Geometry: final body of the model. Coordinates: model frame, mm. Give positions to 0.01 mm unless a question says otherwise; leave off trailing zeros. Loops run counter-clockwise (first coordinate to the right, second up) from the corner with the lowest first, then second, coordinate; pieces in that order, holes last. Notation, with made-up numbers: (81, 53) -> (133, 53) arc R31 ccw to (133, 81) -> close; hole circle Ø1 at (58, -35.75). An arc over 180 degrees is marked (long way). One line per question, with ' | ' between items. Start each with the question number.
Item 1: Section D-D on z = -2.5. Return loops of the section in (x, y), then the cut area to 3 significant figures.
Item 2: Material intervals for line 1 along Y through (x, z) = (0, -2.4); line 2 along X through (y, z) = (2.5, -0.05); line 3 along X through (y, z) = (1, -0.35), sorted ascending. Write a range as [from, to].
Item 3: Section C-C on z = -0.25. Return loops of the section in (x, y).
Item 4: Pin query (flat end, axial travel): P1, Ø2.5, axis at x = 14, y = 0, coming from the -Z side. Return the tip coordinate at first contact, or that it passes through.
Item 5: Section B-B on x = 18. Return loops of the section in (y, z), then the cut area to 3 significant figures.
Item 6: Mould query, pull axis Y, two halves, no side actions, for faces 1 (the flat face through (21, 0, -1)), 2 (the cylindrical face through (16.62, 0.44, -1.52)), 3 (the cylindrical face through (-2.715, -3.699, -1.521)), 4 (the cylindrical face through (12.661, -0.555, -1.521)). Classes: released by +Y, released by -Y, zero draft, split by the parting line, or undercut.
Item 7: Section A-A on y = -1. Return loops of the section in (x, z).
from build123d import *

# Parameters (mm, degrees)
F0_W     = 6
F0_H     = 8
F0_W_2   = 12
F1_DEPTH = 3
F2_D     = 2.9
F4_D     = 2.3
F5_R     = 1


with BuildPart() as f1:
    # F0 (on Top) → F1 (new body)
    with BuildSketch(Plane.XY):
        Rectangle(F0_W, F0_H)
        with Locations((9, 0)):
            Rectangle(F0_W_2, F0_H)
        with Locations((18, 0)):
            Rectangle(F0_W, F0_H)
    extrude(amount=-F1_DEPTH)

    # F2 (through all)
    with Locations(Plane.XY):
        with Locations((0, 0), (4, 0), (14, 0), (18, 0)):
            Hole(F2_D / 2)

    # F4 (through all)
    with Locations(Plane.XZ.offset(4)):
        with Locations((9, 0)):
            Hole(F4_D / 2)

    # F5
    f5_edges = [f1.edges().sort_by_distance(p)[0] for p in [
        (-3, -4, -1.5),
        (21, -4, -1.5),
        (21, 4, -1.5),
        (-3, 4, -1.5),
    ]]
    fillet(f5_edges, radius=F5_R)


solid = f1.part
Result sheet:
1) outline: (-3, -3) arc R1 ccw to (-2, -4) -> (20, -4) arc R1 ccw to (21, -3) -> (21, 3) arc R1 ccw to (20, 4) -> (-2, 4) arc R1 ccw to (-3, 3) -> close; hole circle Ø2.9 at (0, 0); hole circle Ø2.9 at (4, 0); hole circle Ø2.9 at (14, 0); hole circle Ø2.9 at (18, 0) | area: 165 mm²
2) line 1: y = [-4, -1.45], [1.45, 4] | line 2: x = [-3, 7.85], [10.15, 21] | line 3: x = [-3, -1.05], [1.05, 2.95], [5.05, 7.9], [10.1, 12.95], [15.05, 16.95], [19.05, 21]
3) outline: (-3, -3) arc R1 ccw to (-2, -4) -> (7.88, -4) -> (7.88, 4) -> (-2, 4) arc R1 ccw to (-3, 3) -> close; (10.12, -4) -> (20, -4) arc R1 ccw to (21, -3) -> (21, 3) arc R1 ccw to (20, 4) -> (10.12, 4) -> close; hole circle Ø2.9 at (0, 0); hole circle Ø2.9 at (4, 0); hole circle Ø2.9 at (14, 0); hole circle Ø2.9 at (18, 0)
4) P1: passes through
5) outline: (-4, -3) -> (-1.45, -3) -> (-1.45, 0) -> (-4, 0) -> close; (1.45, -3) -> (4, -3) -> (4, 0) -> (1.45, 0) -> close | area: 15.3 mm²
6) face 1: zero draft | face 2: undercut | face 3: released by -Y | face 4: undercut
7) outline: (-3, -3) -> (-1.05, -3) -> (-1.05, 0) -> (-3, 0) -> close; (1.05, -3) -> (2.95, -3) -> (2.95, 0) -> (1.05, 0) -> close; (5.05, -3) -> (12.95, -3) -> (12.95, 0) -> (10.15, 0) arc R1.15 cw to (7.85, 0) -> (5.05, 0) -> close; (15.05, -3) -> (16.95, -3) -> (16.95, 0) -> (15.05, 0) -> close; (19.05, -3) -> (21, -3) -> (21, 0) -> (19.05, 0) -> close
